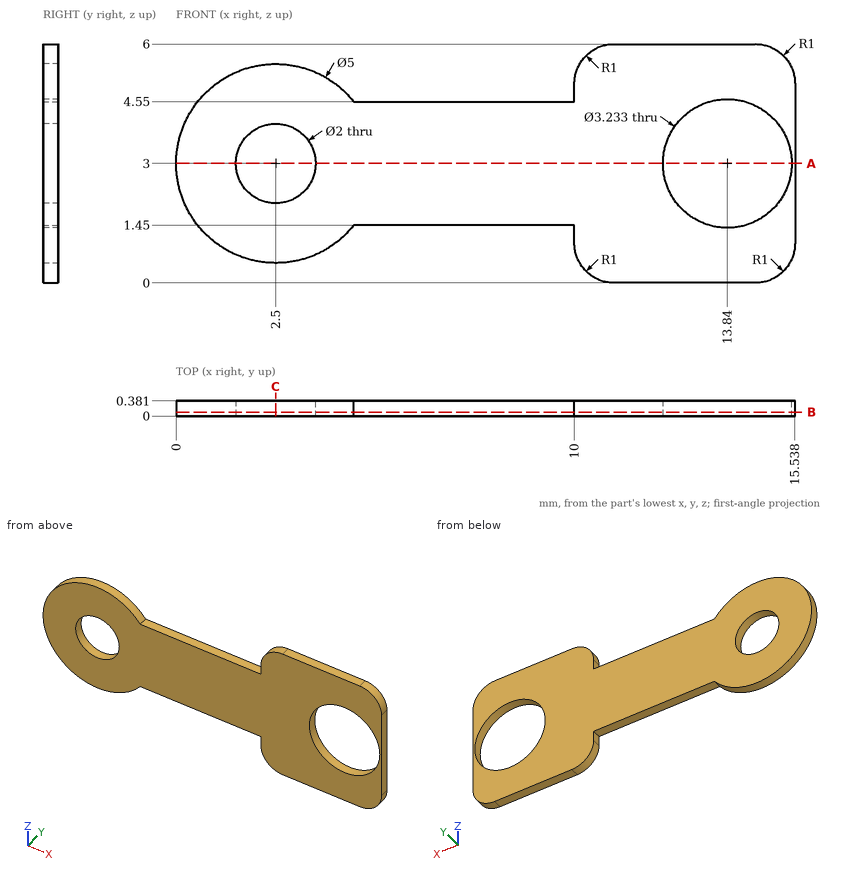
Study the drawing (mm; zero at the part's minimum x, y, z) and answer. Give positions to 0.01 mm unless a question says otherwise; leave off trailing zeros. Loops run counter-clockwise (first coordinate to the right, second up) from the corner with the lowest first, then second, coordinate; pieces in that order, holes last. Notation, with made-up numbers: (86.5, -27) -> (99.5, -27) arc R20 cw to (99.5, -20) -> close; hole circle Ø8 at (53, 41). An arc over 180 degrees is marked (long way). Use a Markdown table: item, result. Add a question column.
1) This flat-tipped pin is pushed along its axis until it touches: P1, Ø1.6, axis at x = 2.5, z = 3, coming from the +Y side. Where does it stop, or does it pass through?
2) The part is cut by section B-B, the plane y = 0.1. Determine the outline of the cut face in (x, z).
3) The part is cut by section A-A, the plane z = 3. Determine the outline of the cut face in (x, y).
4) The part is cut by section C-C, the plane x = 2.5. Determine the outline of the cut face in (y, z).
5) Consider line 1 along X through (y, z) = (0.2, 1) (1 decimal); line 2 along Z through (x, y) = (2.5, 0.35); line 3 along Z through (x, y) = (12.5, 0.15) (1 decimal). Determine where each line is inside the solid, lowest interval first.
Reported:
| question | item | result |
|---|---|---|
| 1 | P1 | passes through |
| 2 | outline | (4.46, 1.45) -> (10, 1.45) -> (10, 1) arc R1 ccw to (11, 0) -> (14.54, 0) arc R1 ccw to (15.54, 1) -> (15.54, 5) arc R1 ccw to (14.54, 6) -> (11, 6) arc R1 ccw to (10, 5) -> (10, 4.55) -> (4.46, 4.55) arc R2.5 ccw (long way) to start; hole circle Ø2 at (2.5, 3); hole circle Ø3.23 at (13.84, 3) |
| 3 | outline | (0, 0) -> (1.5, 0) -> (1.5, 0.38) -> (0, 0.38) -> close; (3.5, 0) -> (12.22, 0) -> (12.22, 0.38) -> (3.5, 0.38) -> close; (15.46, 0) -> (15.54, 0) -> (15.54, 0.38) -> (15.46, 0.38) -> close |
| 4 | outline | (0, 0.5) -> (0.38, 0.5) -> (0.38, 2) -> (0, 2) -> close; (0, 4) -> (0.38, 4) -> (0.38, 5.5) -> (0, 5.5) -> close |
| 5 | line 1 | x = 1 to 4, 10 to 15.5 |
| 5 | line 2 | z = 0.5 to 2, 4 to 5.5 |
| 5 | line 3 | z = 0 to 2.1, 3.9 to 6 |
